```python
from build123d import *

# Parameters (mm, degrees)
SKETCH1_W               = 130
SKETCH1_H               = 80
SKETCH1_R               = 3
SKETCH1_W_2             = 12
SKETCH1_H_2             = 46
BOSS_EXTRUDE1_DEPTH     = 5
FILLET1_R               = 2
SKETCH2_W               = 130
SKETCH2_H               = 5
BOSS_EXTRUDE2_DEPTH     = 70
SKETCH3_W               = 5
SKETCH3_H               = 70
BOSS_EXTRUDE3_DEPTH     = 75
CUT_EXTRUDE1_DEPTH      = 129.452325787
CUT_EXTRUDE1_DEPTH_BACK = 129.452325787
SKETCH4_R               = 6
SKETCH4_R_2             = 2.5


with BuildPart() as part:
    # Sketch1 → Boss-Extrude1 (new body)
    with BuildSketch(Plane(origin=(0, 0, 0), x_dir=(1, 0, 0), z_dir=(0, 1, 0))):
        Rectangle(SKETCH1_W, SKETCH1_H)
        with Locations(Location((-14.35, 0, 0), (0, 0, 270))):
            Circle(SKETCH1_R, mode=Mode.SUBTRACT)
        with Locations(Location((-55.65, 0, 0), (0, 0, 270))):
            Circle(SKETCH1_R, mode=Mode.SUBTRACT)
        with Locations(Location((55.65, 0, 0), (0, 0, 90))):
            Circle(SKETCH1_R, mode=Mode.SUBTRACT)
        with Locations(Location((14.35, 0, 0), (0, 0, 90))):
            Circle(SKETCH1_R, mode=Mode.SUBTRACT)
        Rectangle(SKETCH1_W_2, SKETCH1_H_2, mode=Mode.SUBTRACT)
    extrude(amount=BOSS_EXTRUDE1_DEPTH)

    # Fillet1
    fillet1_edges = [part.edges().sort_by_distance(p)[0] for p in [
        (-6, 2.5, -23),
        (-6, 2.5, 23),
        (6, 2.5, 23),
        (6, 2.5, -23),
    ]]
    fillet(fillet1_edges, radius=FILLET1_R)

    # Sketch2 → Boss-Extrude2 (add)
    with BuildSketch(Plane.XZ):
        with Locations((0, -37.5)):
            Rectangle(SKETCH2_W, SKETCH2_H)
    extrude(amount=BOSS_EXTRUDE2_DEPTH)

    # Sketch3 → Boss-Extrude3 (add)
    with BuildSketch(Plane.XY.offset(-35)):
        with Locations((-32.5, -35)):
            Rectangle(SKETCH3_W, SKETCH3_H)
        with Locations((32.5, -35)):
            Rectangle(SKETCH3_W, SKETCH3_H)
    extrude(amount=BOSS_EXTRUDE3_DEPTH)

    # Sketch4 → Cut-Extrude1 (cut, two sides: drawn at the far end of the back side and taken through both)
    with BuildSketch(Plane.ZY.offset(35).offset(-CUT_EXTRUDE1_DEPTH_BACK)):
        with Locations(Location((0, -35, 0), (0, 0, 270))):
            Circle(SKETCH4_R)
        with Locations(Location((0, -16.5, 0), (0, 0, 270))):
            Circle(SKETCH4_R_2)
        with Locations(Location((0, -53.5, 0), (0, 0, 270))):
            Circle(SKETCH4_R_2)
    extrude(amount=CUT_EXTRUDE1_DEPTH + CUT_EXTRUDE1_DEPTH_BACK, mode=Mode.SUBTRACT)


solid = part.part
```
Work out the finished part from the listing and answer in its coordinate system (mm). A direction names the side the tool comes from. Give positions to 0.01 mm unless a question says otherwise; leave off trailing zeros. Order: outer loops, then holes, each group sorted by start corner. A loop starts at its lowest first (then second) coordinate and runs counter-clockwise, first axis right, second up.
1. Each of these flat-tipped pins is pushed along its axis until it touches: P1, Ø10, axis at x = 20, z = 22.5, coming from the -Y side; P2, Ø3, axis at x = 21, y = -15.5, coming from the +Z side; P3, Ø14, axis at y = -35, z = 0, coming from the +X side. Where does it stop, or does it pass through?
Result sheet:
P1: stops at y = 0
P2: stops at z = -35
P3: stops at x = 35
2. Section A-A, the plane y = -16.5 is taken. Determine the outline of the cut face in (x, z), and give its area (3 significant figures).
Result sheet:
outline: (-65, -40) - (65, -40) - (65, -35) - (35, -35) - (35, -2.5) - (30, -2.5) - (30, -35) - (-30, -35) - (-30, -2.5) - (-35, -2.5) - (-35, -35) - (-65, -35) - close; (-35, 2.5) - (-30, 2.5) - (-30, 40) - (-35, 40) - close; (30, 2.5) - (35, 2.5) - (35, 40) - (30, 40) - close
area: 1,350 mm2
3. Straight lines are drawn through the part: L1, parallel to Y at x = 33, z = 0; L2, parallel to X at y = -8, z = -22; L3, parallel to Z at x = 33.8, y = -16.5. For each, find the intervals that lie inside material, in ascending order.
Result sheet:
L1: y = -70 to -56, -51 to -41, -29 to -19, -14 to 5
L2: x = -35 to -30, 30 to 35
L3: z = -40 to -2.5, 2.5 to 40
4. Section B-B, the plane x = 55.65 is taken. Determine the outline of the cut face in (y, z), and give its area (3 significant figures).
Result sheet:
outline: (-70, -40) - (5, -40) - (5, -3) - (0, -3) - (0, -35) - (-70, -35) - close; (0, 3) - (5, 3) - (5, 40) - (0, 40) - close
area: 720 mm2
5. The mould has two halves that part along Y. Classify faces 1 (the flat face through (-15, 5, 8)), 2 (the flat face through (-0.3, -70, -35.4)), 3 (the cylindrical face through (33, -14, 0)), 4 (the flat face through (-6, 2, 0)): released by +Y, released by -Y, zero draft, split by the parting line, or undercut.
Result sheet:
face 1: released by +Y
face 2: released by -Y
face 3: undercut
face 4: zero draft
6. Section D-D, the plane x = 32.5 is taken. Determine the outline of the cut face in (y, z).
Result sheet:
outline: (-70, -40) - (5, -40) - (5, 40) - (-70, 40) - close; hole circle Ø5 at (-53.5, 0); hole circle Ø12 at (-35, 0); hole circle Ø5 at (-16.5, 0)
7. Section C-C, the plane z = -8 is taken. Determine the outline of the cut face in (x, y).
Result sheet:
outline: (-65, 0) - (-35, 0) - (-35, -70) - (-30, -70) - (-30, 0) - (-6, 0) - (-6, 5) - (-65, 5) - close; (6, 0) - (30, 0) - (30, -70) - (35, -70) - (35, 0) - (65, 0) - (65, 5) - (6, 5) - close
8. For faces 5 (the flat face through (35, -43, 2)), 6 (the flat face through (6, 2, 0)), 7 (the flat face through (0, 1, 40)), 8 (the cylindrical face through (-32.47, -55.81, -0.96)), 9 (the flat face through (-7, 0, 2)), determine the directions among +Z, -Z, +X, -X, +Y, -Y from which every point of the face is accessible in a straight line to the end or side of a thin tool.
Result sheet:
face 5: +Z, +X, -Y
face 6: +Y, -Y
face 7: +Z, +X, -X, +Y, -Y
face 8: +X, -X
face 9: +Z, -Y
